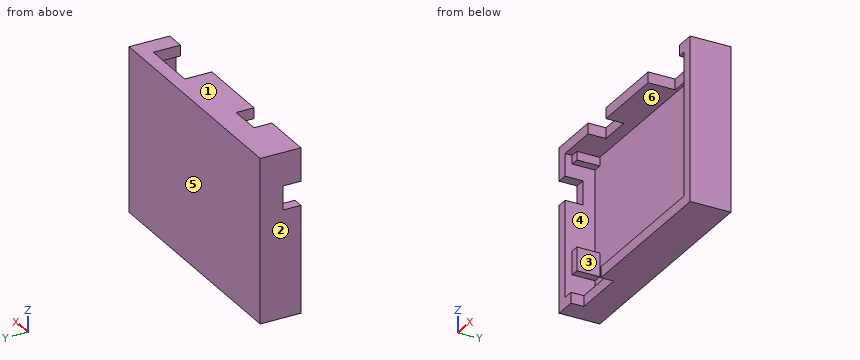
from build123d import *

# Parameters (mm, degrees)
SKETCH1_W           = 33
SKETCH1_H           = 23
SKETCH1_W_2         = 30
SKETCH1_H_2         = 20
BOSS_EXTRUDE1_DEPTH = 5.7
SKETCH2_W           = 30
SKETCH2_H           = 20
BOSS_EXTRUDE2_DEPTH = 1.5
CUT_EXTRUDE1_REACH  = 25
SKETCH3_W           = 7.5
SKETCH3_H           = 3.6
CUT_EXTRUDE2_REACH  = 25
SKETCH4_W           = 7.9
SKETCH4_H           = 7.6
SKETCH4_W_2         = 4.5
SKETCH4_H_2         = 5
CUT_EXTRUDE3_REACH  = 35
SKETCH5_W           = 3.35
SKETCH5_H           = 5
SKETCH6_W           = 2
SKETCH6_H           = 12.5
BOSS_EXTRUDE3_DEPTH = 2.2
SKETCH7_W           = 1.2
SKETCH7_H           = 3.3
SKETCH7_H_2         = 1.2
BOSS_EXTRUDE4_DEPTH = 3.2


with BuildPart() as part:
    # Sketch1 → Boss-Extrude1 (new body)
    with BuildSketch(Plane(origin=(0, 0, 0), x_dir=(1, 0, 0), z_dir=(0, 1, 0))):
        Rectangle(SKETCH1_W, SKETCH1_H)
        Rectangle(SKETCH1_W_2, SKETCH1_H_2, mode=Mode.SUBTRACT)
    extrude(amount=BOSS_EXTRUDE1_DEPTH)

    # Sketch2 → Boss-Extrude2 (add)
    with BuildSketch(Plane(origin=(0, 5.7, 0), x_dir=(1, 0, 0), z_dir=(0, 1, 0))):
        Rectangle(SKETCH2_W, SKETCH2_H)
    extrude(amount=-BOSS_EXTRUDE2_DEPTH)

    # Sketch3 → Cut-Extrude1 (cut, up to next)
    with BuildSketch(Plane(origin=(0, 0, -11.5), x_dir=(-1, 0, 0), z_dir=(0, 0, -1)), mode=Mode.PRIVATE) as cut_extrude1_sk1:
        with Locations((9.75, 0)):
            Rectangle(SKETCH3_W, SKETCH3_H)
    cut_extrude1_tool1 = extrude(cut_extrude1_sk1.sketch, amount=-CUT_EXTRUDE1_REACH, mode=Mode.PRIVATE) & part.part
    add(cut_extrude1_tool1.solids().sort_by_distance((-9.75, 0, -11.5))[0], mode=Mode.SUBTRACT)

    # Sketch4 → Cut-Extrude2 (cut, up to next)
    with BuildSketch(Plane.XY.offset(11.5), mode=Mode.PRIVATE) as cut_extrude2_sk1:
        with Locations((9.85, 0)):
            Rectangle(SKETCH4_W, SKETCH4_H)
    cut_extrude2_tool1 = extrude(cut_extrude2_sk1.sketch, amount=-CUT_EXTRUDE2_REACH, mode=Mode.PRIVATE) & part.part
    add(cut_extrude2_tool1.solids().sort_by_distance((9.85, 0, 11.5))[0], mode=Mode.SUBTRACT)
    # Sketch4 → Cut-Extrude2 (cut, up to next)
    with BuildSketch(Plane.XY.offset(11.5), mode=Mode.PRIVATE) as cut_extrude2_sk2:
        with Locations((-6.95, 0)):
            Rectangle(SKETCH4_W_2, SKETCH4_H_2)
    cut_extrude2_tool2 = extrude(cut_extrude2_sk2.sketch, amount=-CUT_EXTRUDE2_REACH, mode=Mode.PRIVATE) & part.part
    add(cut_extrude2_tool2.solids().sort_by_distance((-6.95, 0, 11.5))[0], mode=Mode.SUBTRACT)

    # Sketch5 → Cut-Extrude3 (cut, up to next)
    with BuildSketch(Plane.ZY.offset(16.5), mode=Mode.PRIVATE) as cut_extrude3_sk1:
        with Locations((5.175, 0)):
            Rectangle(SKETCH5_W, SKETCH5_H)
    cut_extrude3_tool1 = extrude(cut_extrude3_sk1.sketch, amount=-CUT_EXTRUDE3_REACH, mode=Mode.PRIVATE) & part.part
    add(cut_extrude3_tool1.solids().sort_by_distance((-16.5, 0, 5.175))[0], mode=Mode.SUBTRACT)

    # Sketch6 → Boss-Extrude3 (add)
    with BuildSketch(Plane.XZ.offset(-4.2)):
        with Locations((14, -3.75)):
            Rectangle(SKETCH6_W, SKETCH6_H)
    extrude(amount=BOSS_EXTRUDE3_DEPTH)

    # Sketch7 → Boss-Extrude4 (add)
    with BuildSketch(Plane.XZ.offset(-4.2)):
        with Locations((-14.4, -4.95)):
            Rectangle(SKETCH7_W, SKETCH7_H)
        with Locations((-14.4, 9.4)):
            Rectangle(SKETCH7_W, SKETCH7_H_2)
    extrude(amount=BOSS_EXTRUDE4_DEPTH)


solid = part.part
Here's how the part is built. I have some questions about the finished solid (model axes, mm). Face numbers are marked on the shaded views. A direction names the side the tool comes from. Round coordinates to 2 decimals unless told otherwise and drop trailing zeros. Order: outer loops, then holes, each group sorted by start corner. A loop starts at its lowest first (then second) coordinate and runs counter-clockwise, first axis right, second up. Notation, with made-up numbers: (19.5, 51.5) -> (27.5, 51.5) arc R18 cw to (27.5, 60.5) -> close; hole circle Ø1 at (-13, -39). An arc over 180 degrees is marked (long way). Return JSON: item names as keys, results as strings.
Q1. I need wall thicknesses on line 1 along Z through (x, y) = (-14, 2.1); line 2 along X through (y, z) = (1.3, 2.5); line 3 along X through (y, z) = (3.65, 10.75). Which ranges of each line are inside material? Lowest first, please. Write a range as from..to.
Filled sheet:
{"line 1": "z = -11.5..-10, -6.6..-3.3, 8.8..11.5", "line 2": "x = -16.5..-15, 15..16.5", "line 3": "x = -16.5..5.9, 13.8..16.5"}
Q2. For pin 1 Ø0.8 at (x, z) = (-8.5, -10.5) entering from -Y; pin 2 Ø4 at (x, z) = (0.5, -0.5) entering from -Y; pin 3 Ø1.6 at (x, z) = (-8, 10.5) entering from -Y, each with a flat end and sliding along its axis, tell me the tip position at first contact or that it passes through.
Filled sheet:
{"pin 1": "stops at y = 1.8", "pin 2": "stops at y = 4.2", "pin 3": "stops at y = 2.5"}
Q3. If we section it at B-B on z = 7.5: List the corners of the cut face in (x, y) for me, plus the area to 3 significant figures.
Filled sheet:
{"outline": "(-16.5, 0) -> (-15, 0) -> (-15, 4.2) -> (15, 4.2) -> (15, 0) -> (16.5, 0) -> (16.5, 5.7) -> (-16.5, 5.7) -> close", "area": "62.1 mm^2"}
Q4. If we section it at D-D on z = 0: List the corners of the cut face in (x, y) for me.
Filled sheet:
{"outline": "(-16.5, 0) -> (-15, 0) -> (-15, 4.2) -> (13, 4.2) -> (13, 2) -> (15, 2) -> (15, 0) -> (16.5, 0) -> (16.5, 5.7) -> (-16.5, 5.7) -> close"}
Q5. If we mould it in two halves opening along Z, with no side actions, what happens to the marked faces 1, 2, 3 and 4? For each: released by +Z, released by -Z, zero draft, split by the parting line, or undercut.
Filled sheet:
{"face 1": "released by +Z", "face 2": "zero draft", "face 3": "undercut", "face 4": "undercut"}
Q6. If we section it at C-C on z = -4.5: List the corners of the cut face in (x, y) for me.
Filled sheet:
{"outline": "(-16.5, 0) -> (-15, 0) -> (-15, 1) -> (-13.8, 1) -> (-13.8, 4.2) -> (13, 4.2) -> (13, 2) -> (15, 2) -> (15, 0) -> (16.5, 0) -> (16.5, 5.7) -> (-16.5, 5.7) -> close"}
Q7. If we section it at A-A on x = -8: List the corners of the cut face in (y, z) for me, plus the area to 4 significant figures.
Filled sheet:
{"outline": "(1.8, -11.5) -> (5.7, -11.5) -> (5.7, 11.5) -> (2.5, 11.5) -> (2.5, 10) -> (4.2, 10) -> (4.2, -10) -> (1.8, -10) -> close", "area": "40.65 mm^2"}
Q8. Which directions (+Z, -Z, +X, -X, +Y, -Y) give clear straight access to the entire face, cutting with the end or side of a thin tool? Please do the marked faces 5 and 6.
Filled sheet:
{"face 5": "+Z, -Z, +X, -X, +Y", "face 6": "-Y"}
